Design review of the part built by this model. Coordinates are the model's own, in mm. Face numbers are marked on the shaded views. A direction names the side the tool comes from. Give positions to 0.01 mm unless a question says otherwise; leave off trailing zeros. Write each loop counter-clockwise with the first axis right and the second up, starting at its lowest first coordinate (ties: lowest second). Pieces come first, ordered by that corner, then holes. Notation, with made-up numbers: (-33.75, 58.25) - (4.25, 58.25) arc R10 cw to (4.25, 64.25) - close; hole circle Ø6 at (44, -6). An arc over 180 degrees is marked (long way). Use a Markdown table: item, result. Add a question column.
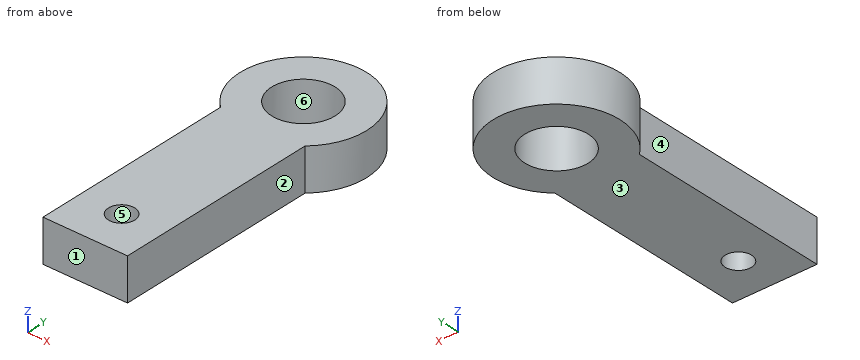
```python
from build123d import *

# Parameters (mm, degrees)
HORN_ARM_SKETCH_W       = 8
HORN_ARM_SKETCH_H       = 24
HORN_ARM_DEPTH          = 4
HORN_HUB_SKETCH_R       = 6
HORN_HUB_DEPTH          = 4
SHAFT_BORE_SKETCH_R     = 3
SHAFT_BORE_DEPTH        = 4
BALL_STUD_HOLE_SKETCH_R = 1.25
BALL_STUD_HOLE_DEPTH    = 4


with BuildPart() as part:
    # Horn Arm Sketch → Horn Arm (new body)
    with BuildSketch(Plane.XY.offset(13.2)):
        with Locations((-91, 71.4)):
            Rectangle(HORN_ARM_SKETCH_W, HORN_ARM_SKETCH_H)
    extrude(amount=HORN_ARM_DEPTH)

    # Horn Hub Sketch → Horn Hub (add)
    with BuildSketch(Plane.XY.offset(13.2)):
        with Locations((-91, 83.4)):
            Circle(HORN_HUB_SKETCH_R)
    extrude(amount=HORN_HUB_DEPTH)

    # Shaft Bore Sketch → Shaft Bore (cut)
    with BuildSketch(Plane.XY.offset(13.2)):
        with Locations((-91, 83.4)):
            Circle(SHAFT_BORE_SKETCH_R)
    extrude(amount=SHAFT_BORE_DEPTH, mode=Mode.SUBTRACT)

    # Ball Stud Hole Sketch → Ball Stud Hole (cut)
    with BuildSketch(Plane.XY.offset(13.2)):
        with Locations((-91, 63.4)):
            Circle(BALL_STUD_HOLE_SKETCH_R)
    extrude(amount=BALL_STUD_HOLE_DEPTH, mode=Mode.SUBTRACT)


solid = part.part
```
(1) Mouldability with a two-part tool opening along X and no side actions: class the marked faces 3, 4, 5 and 6 as +X half, -X half, draft (parallel to the pull), parting line (faces both ways), or undercut.
(2) Add section B-B (x = -91). State the section outline as (y, z) points.
(3) Add section D-D (x = -93.5). State the section outline as (y, z) points, and give its area (3 significant figures).
(4) Tool access review of the marked faces 1 and 2: name each direction out of +Z, -Z, +X, -X, +Y, -Y from which nothing blocks a thin tool from reaching the whole face with its end or side.
(5) Insertion check: pin 1 (2 mm diameter, centred on y = 71, z = 15.5, fed in from -X); pin 2 (2 mm diameter, centred on x = -91, y = 63.4, fed in from -Z); pin 3 (2 mm diameter, centred on y = 66, z = 14.5, fed in from +X); pin 4 (1 mm diameter, centred on x = -93, z = 16.5, fed in from +Y). Each pin has a flat end and moves straight along its axis. Give the tip position at first contact, or say it passes through.
(6) Add section A-A (y = 83.4). State the section outline as (x, z) points.
(7) Add section C-C (z = 15.1). State the section outline as (x, y) points.
(8) For line 1 along Y through (x, z) = (-91, 15.95); line 2 along X through (y, z) = (65, 15.95); line 3 along Y through (x, z) = (-89, 16.45), list the stretches that pass through material, from the lowest coordinate up.
Answers follow:
| question | item | result |
|---|---|---|
| 1 | face 3 | draft |
| 1 | face 4 | -X half |
| 1 | face 5 | undercut |
| 1 | face 6 | undercut |
| 2 | outline | (59.4, 13.2) - (62.15, 13.2) - (62.15, 17.2) - (59.4, 17.2) - close; (64.65, 13.2) - (80.4, 13.2) - (80.4, 17.2) - (64.65, 17.2) - close; (86.4, 13.2) - (89.4, 13.2) - (89.4, 17.2) - (86.4, 17.2) - close |
| 3 | outline | (59.4, 13.2) - (81.74, 13.2) - (81.74, 17.2) - (59.4, 17.2) - close; (85.06, 13.2) - (88.85, 13.2) - (88.85, 17.2) - (85.06, 17.2) - close |
| 3 | area | 105 mm^2 |
| 4 | face 1 | +Z, -Z, +X, -X, -Y |
| 4 | face 2 | +Z, -Z, +X, -Y |
| 5 | pin 1 | x = -95 |
| 5 | pin 2 | through |
| 5 | pin 3 | x = -87 |
| 5 | pin 4 | y = 89.21 |
| 6 | outline | (-97, 13.2) - (-94, 13.2) - (-94, 17.2) - (-97, 17.2) - close; (-88, 13.2) - (-85, 13.2) - (-85, 17.2) - (-88, 17.2) - close |
| 7 | outline | (-95, 59.4) - (-87, 59.4) - (-87, 78.93) arc R6 ccw (long way) to (-95, 78.93) - close; hole circle Ø6 at (-91, 83.4); hole circle Ø2.5 at (-91, 63.4) |
| 8 | line 1 | 59.4 to 62.15, 64.65 to 80.4, 86.4 to 89.4 |
| 8 | line 2 | -95 to -87 |
| 8 | line 3 | 59.4 to 81.16, 85.64 to 89.06 |
